Geometry: final body of the model. Coordinates: model frame, mm. Face numbers are marked on the shaded views. Coordinates: 2 decimals unless noted, no trailing zeros. Loops run counter-clockwise (first coordinate to the right, second up) from the corner with the lowest first, then second, coordinate; pieces in that order, holes last. Notation, with made-up numbers: (-35, 82) -> (-14, 82) arc R24 ccw to (-14, 115) -> close; hole circle Ø6 at (21, 48). An arc over 180 degrees is marked (long way). One line per item, written item: value. Start each with the question number.
Item 1: Mould query, pull axis Y, two halves, no side actions, for the marked faces 1, 2 and 3. Classes: +Y half, -Y half, draft (parallel to the pull), parting line (faces both ways), or undercut.
Item 2: Section query C-C on z = 4. Return loops of the section in (x, y).
Item 3: Section query D-D on x = 6. Return loops of the section in (y, z), then the cut area to 3 significant figures.
Item 4: Contact query for flat-ended pins moving along their axis: pin 1 Ø3.5 at (x, y) = (0, 0) entering from +Z; pin 2 Ø4 at (y, z) = (-4.5, 6) entering from +X; pin 3 Ø2 at (y, z) = (4, 15.5) entering from +X; pin 4 Ø5.5 at (x, y) = (-1, 1) entering from -Z. Output: stop coordinate, or through.
Item 5: Ray query, probe 1 along Y at (x, z) = (0, 26); probe 2 along Z at (x, y) = (-0.5, 6); probe 3 along Z at (x, y) = (2.25, -0.25). Return the intervals inside material, ascending. Write a range as from..to.
Item 6: Section query A-A on y = 0. Return loops of the section in (x, z).
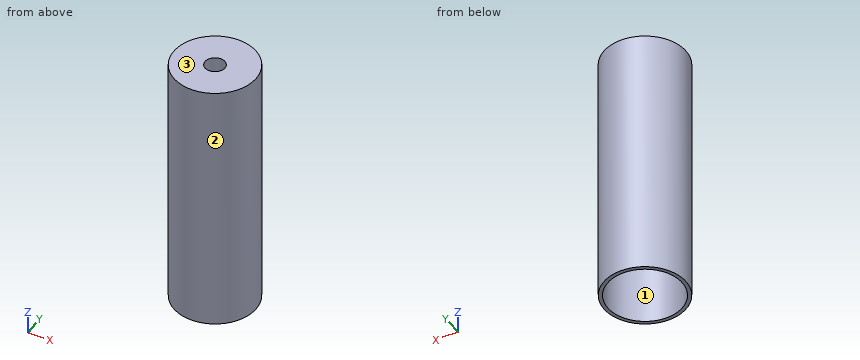
from build123d import *

# Parameters (mm, degrees)
F0_R     = 8.25
F0_R_2   = 7.5
F1_DEPTH = 50
F2_R     = 8.25
F3_DEPTH = 1.5
F4_R     = 2
F5_DEPTH = 25
F6_R     = 3.5
F6_R_2   = 2
F7_DEPTH = 5


with BuildPart() as f1:
    # F0 (on Top) → F1 (new body)
    with BuildSketch(Plane.XY):
        Circle(F0_R)
        Circle(F0_R_2, mode=Mode.SUBTRACT)
    extrude(amount=F1_DEPTH)

    # F2 (on face) → F3 (join)
    with BuildSketch(Plane.XY.offset(50)):
        Circle(F2_R)
    extrude(amount=F3_DEPTH)

    # F4 (on face) → F5 (cut)
    with BuildSketch(Plane.XY.offset(51.5)):
        Circle(F4_R)
    extrude(amount=-F5_DEPTH, mode=Mode.SUBTRACT)

    # F6 (on face) → F7 (join)
    with BuildSketch(Plane(origin=(0, 0, 50), x_dir=(1, 0, 0), z_dir=(0, 0, -1))):
        Circle(F6_R)
        Circle(F6_R_2, mode=Mode.SUBTRACT)
    extrude(amount=F7_DEPTH)


solid = f1.part
Reply:
1. face 1: undercut
1. face 2: parting line
1. face 3: draft
2. outline: circle Ø16.5 at (0, 0); hole circle Ø15 at (0, 0)
3. outline: (-5.66, 0) -> (-4.5, 0) -> (-4.5, 50) -> (4.5, 50) -> (4.5, 0) -> (5.66, 0) -> (5.66, 51.5) -> (-5.66, 51.5) -> close
3. area: 133 mm²
4. pin 1: passes through
4. pin 2: stops at x = 7.86
4. pin 3: stops at x = 7.69
4. pin 4: stops at z = 45
5. probe 1: y = -8.25..-7.5, 7.5..8.25
5. probe 2: z = 50..51.5
5. probe 3: z = 45..51.5
6. outline: (-8.25, 0) -> (-7.5, 0) -> (-7.5, 50) -> (-3.5, 50) -> (-3.5, 45) -> (-2, 45) -> (-2, 51.5) -> (-8.25, 51.5) -> close; (2, 45) -> (3.5, 45) -> (3.5, 50) -> (7.5, 50) -> (7.5, 0) -> (8.25, 0) -> (8.25, 51.5) -> (2, 51.5) -> close
